```python
from build123d import *

# Parameters (mm, degrees)
F0_R     = 27.4575403643
F1_DEPTH = 152.4
F2_T     = -2.54
F4_D     = 6.35
F4_DEPTH = 12.7
F4_TIP   = 1.9077324654


with BuildPart() as f1:
    # F0 (on Top) → F1 (new body)
    with BuildSketch(Plane.XY):
        with Locations((-34.6127040684, 22.6622130722)):
            Circle(F0_R)
    extrude(amount=F1_DEPTH)

    # F2
    f2_openings = [f1.faces().sort_by_distance(p)[0] for p in [
        (-34.612704, 22.662213, 152.4),
    ]]
    offset(amount=F2_T, openings=f2_openings)

    # F4 (one way)
    with BuildSketch(Plane(origin=(0, 0, 0), x_dir=(1, 0, 0), z_dir=(0, 1, 0))):
        with Locations((-35.1956561208, -44.1724844277)):
            Circle(F4_D / 2)
    extrude(amount=-F4_DEPTH, mode=Mode.SUBTRACT)
    with Locations(Plane(origin=(0, 0, 0), x_dir=(1, 0, 0), z_dir=(0, 1, 0))):
        with Locations((-35.1956561208, -44.1724844277)):
            with Locations((0, 0, -(F4_DEPTH + F4_TIP / 2))):  # 118° drill point
                Cone(0, F4_D / 2, F4_TIP, mode=Mode.SUBTRACT)


solid = f1.part
```
Check sheet for the modelled part. Datum: model origin and axes. Units: mm. A direction names the side the tool comes from. Round coordinates to 2 decimals unless told otherwise and drop trailing zeros. Order: outer loops, then holes, each group sorted by start corner. A loop starts at its lowest first (then second) coordinate and runs counter-clockwise, first axis right, second up. Notation, with made-up numbers: (14.5, 30) - (56.5, 30) arc R17 ccw to (56.5, 47) - close; hole circle Ø10 at (71, -5.75). An arc over 180 degrees is marked (long way). Answer as CSV lines item,"result". Start each with the question number.
1) Section check A-A (x = -17.5). Record the cut outline in (y, z), then the cut area to 3 significant figures.
2) Depth check by flat-ended pin: pin 1 (3 mm diameter, centred on x = -45.5, z = 104.5, fed in from -Y); pin 2 (15 mm diameter, centred on x = -43, y = 27.5, fed in from +Z); pin 3 (4 mm diameter, centred on x = -50, z = 44, fed in from +Y); pin 4 (8.5 mm diameter, centred on x = -35.2, z = 44.17, fed in from -Y). Enter the tip coordinate at first touch or a pass-through.
3) Scan lines: probe 1 along X at (y, z) = (21.5, 23); probe 2 along Z at (x, y) = (-12, 25); probe 3 along X at (y, z) = (39, 66). Record each from-to range of solid material in increasing order.
4) Tool access check on faces 5 (the face through (-35, 23, 0)), 6 (the face through (-37.54, -3.36, 42.03)). Record the directions out of +Z, -Z, +X, -X, +Y, -Y that give a thin tool (end or side, any length) a straight path to the whole face; none if there is none.
5) Section check B-B (y = 46). Record the cut outline in (x, z), then the cut area to 3 significant figures.
6) Section check C-C (z = 29.5). Record the cut outline in (x, y).
7) Draft check along X on faces 1 (the face through (-35, 23, 2.54)), 2 (the face through (-29, -2, 152.4)), 3 (the face through (-8.423, 30.91, 75.133)), 4 (the face through (-23.11, 0.56, 76.42)). Enter one of: +X half, -X half, draft (parallel to the pull), parting line (faces both ways), or undercut.
Determined:
1,outline,"(1.19, 0) - (44.13, 0) - (44.13, 152.4) - (40.77, 152.4) - (40.77, 2.54) - (4.55, 2.54) - (4.55, 152.4) - (1.19, 152.4) - close"
1,area,"1,120 mm^2"
2,pin 1,"y = -3.14"
2,pin 2,"z = 2.54"
2,pin 3,"y = 46.64"
2,pin 4,"y = -4.8"
3,probe 1,"-62.05 to -59.5, -9.72 to -7.18"
3,probe 2,"0 to 2.54"
3,probe 3,"-56.68 to -53.43, -15.8 to -12.54"
4,face 5,"-Z, +X, -X, +Y, -Y"
4,face 6,"-Y"
5,outline,"(-49.08, 0) - (-20.15, 0) - (-20.15, 152.4) - (-25.88, 152.4) - (-25.88, 2.54) - (-43.34, 2.54) - (-43.34, 152.4) - (-49.08, 152.4) - close"
5,area,"1,790 mm^2"
6,outline,"circle Ø54.92 at (-34.61, 22.66); hole circle Ø49.84 at (-34.61, 22.66)"
7,face 1,"undercut"
7,face 2,"draft"
7,face 3,"parting line"
7,face 4,"undercut"
